Print and shaded views of the part. All mm, measured from the part's lowest x, y and z. Coordinates: 2 decimals unless noted, no trailing zeros. Order: outer loops, then holes, each group sorted by start corner. A loop starts at its lowest first (then second) coordinate and runs counter-clockwise, first axis right, second up. Notation, with made-up numbers: M -27.5,80.5 L 21.5,80.5 A9 cw 21.5,89.5 Z; hole C 9,45.25 d11. An arc over 180 degrees is marked long. One line per item, written item: value.
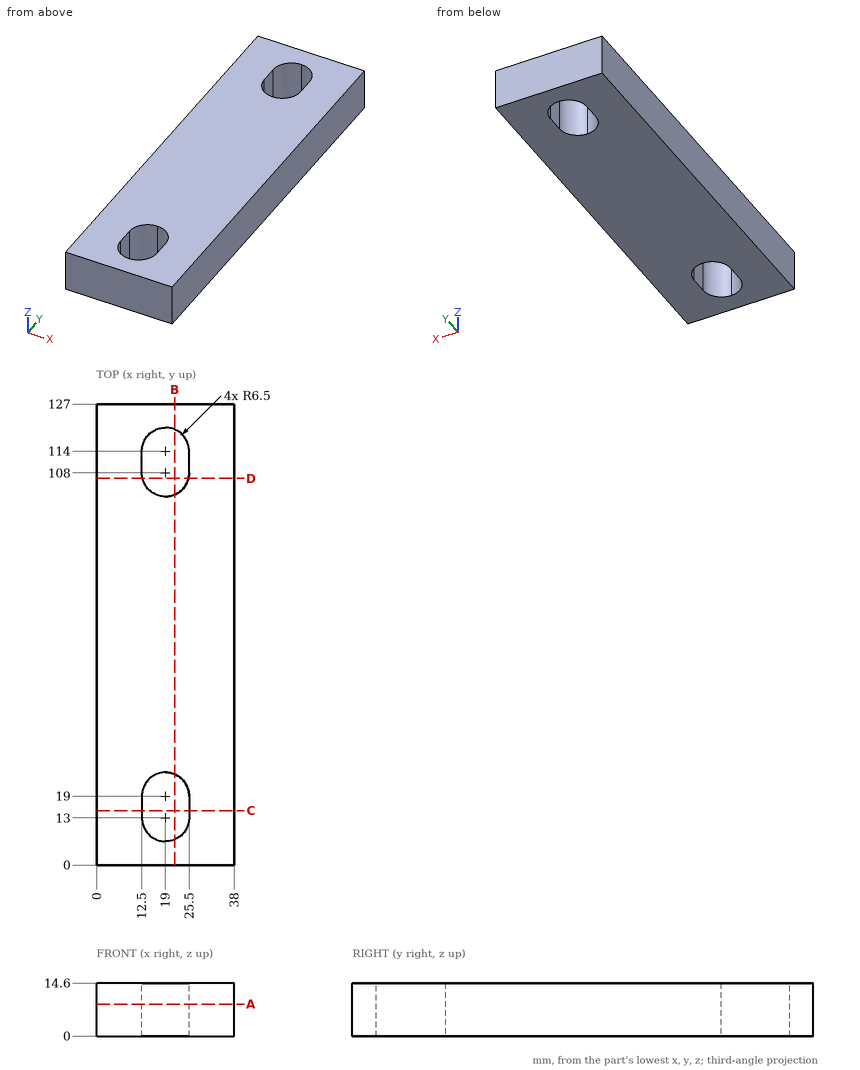
Q1. Drill centre lines: line 1 along X through (y, z) = (18, 0.5); line 2 along Y through (x, z) = (24, 1.75); line 3 along Y through (x, z) = (15, 8.75). Where is each one in solid material? Low to high.
Recorded:
line 1: x = 0 to 12.5, 25.5 to 38
line 2: y = 0 to 8.85, 23.15 to 103.85, 118.15 to 127
line 3: y = 0 to 7.88, 24.12 to 102.88, 119.12 to 127
Q2. Slice it at D-D (y = 106.5). List the corners of the cut face in (x, z).
Recorded:
outline: M 0,0 L 12.68,0 L 12.68,14.6 L 0,14.6 Z; M 25.32,0 L 38,0 L 38,14.6 L 25.32,14.6 Z
Q3. Slice it at C-C (y = 15). List the corners of the cut face in (x, z).
Recorded:
outline: M 0,0 L 12.5,0 L 12.5,14.6 L 0,14.6 Z; M 25.5,0 L 38,0 L 38,14.6 L 25.5,14.6 Z
Q4. Slice it at A-A (z = 8.75). List the corners of the cut face in (x, y).
Recorded:
outline: M 0,0 L 38,0 L 38,127 L 0,127 Z; hole M 12.5,13 A6.5 ccw 25.5,13 L 25.5,19 A6.5 ccw 12.5,19 Z; hole M 12.5,108 A6.5 ccw 25.5,108 L 25.5,114 A6.5 ccw 12.5,114 Z
Q5. Slice it at B-B (x = 21.5). List the corners of the cut face in (y, z).
Recorded:
outline: M 0,0 L 7,0 L 7,14.6 L 0,14.6 Z; M 25,0 L 102,0 L 102,14.6 L 25,14.6 Z; M 120,0 L 127,0 L 127,14.6 L 120,14.6 Z
